Input: part model. Units: mm. Frame: model coordinates. A direction names the side the tool comes from. Coordinates: 2 decimals unless noted, no trailing zeros. Write each loop counter-clockwise with the first axis right and the second up, starting at its lowest first coordinate (ties: lowest second). Pieces come first, ordered by that corner, then holes.
from build123d import *

# Parameters (mm, degrees)
SKETCH1_W               = 40
SKETCH1_H               = 102
BOSS_EXTRUDE1_DEPTH     = 8.5
SKETCH2_W               = 35
SKETCH2_H               = 70
CUT_EXTRUDE1_DEPTH      = 3
SKETCH3_W               = 10.5
SKETCH3_H               = 10
CUT_EXTRUDE2_DEPTH      = 1.35
SKETCH4_W               = 12.5
SKETCH4_H               = 6
CUT_EXTRUDE3_DEPTH      = 3.1
SKETCH5_W               = 8.5
SKETCH5_H               = 17.5
PCB_PLACE_DEPTH         = 3.1
SKETCH6_W               = 8.5
SKETCH6_H               = 1.6
NICKEL_STRIP_HOLE_DEPTH = 66.369411807
CUT_EXTRUDE4_REACH      = 67.698
SKETCH7_W               = 8.5
SKETCH7_H               = 17.5
SKETCH8_W               = 8.5
SKETCH8_H               = 1.6
CUT_EXTRUDE5_DEPTH      = 10
SKETCH9_W               = 8.5
SKETCH9_H               = 102
NICKEL_STRIP_RAIL_DEPTH = 2.5
FILLET3_R               = 2.325
FILLET4_RADIUS          = 1.45
FILLET4_LENGTH          = 8.5


with BuildPart() as part:
    # Sketch1 → Boss-Extrude1 (new body)
    with BuildSketch(Plane(origin=(0, 0, 0), x_dir=(1, 0, 0), z_dir=(0, 1, 0))):
        with Locations((0, 11)):
            Rectangle(SKETCH1_W, SKETCH1_H)
    extrude(amount=BOSS_EXTRUDE1_DEPTH)

    # Sketch2 → Cut-Extrude1 (cut)
    with BuildSketch(Plane(origin=(0, 8.5, 0), x_dir=(1, 0, 0), z_dir=(0, 1, 0))):
        with Locations((0, -2)):
            Rectangle(SKETCH2_W, SKETCH2_H)
    extrude(amount=-CUT_EXTRUDE1_DEPTH, mode=Mode.SUBTRACT)

    # Sketch3 → Cut-Extrude2 (cut)
    with BuildSketch(Plane(origin=(0, 8.5, 0), x_dir=(1, 0, 0), z_dir=(0, 1, 0))):
        with Locations((-6.65, 38)):
            Rectangle(SKETCH3_W, SKETCH3_H)
        with Locations((6.65, 38)):
            Rectangle(SKETCH3_W, SKETCH3_H)
    extrude(amount=-CUT_EXTRUDE2_DEPTH, mode=Mode.SUBTRACT)

    # Sketch4 → Cut-Extrude3 (cut)
    with BuildSketch(Plane(origin=(0, 8.5, 0), x_dir=(1, 0, 0), z_dir=(0, 1, 0))):
        with Locations((6.65, 40)):
            Rectangle(SKETCH4_W, SKETCH4_H)
    extrude(amount=-CUT_EXTRUDE3_DEPTH, mode=Mode.SUBTRACT)

    # Sketch5 → PCB place (cut)
    with BuildSketch(Plane(origin=(0, 8.5, 0), x_dir=(1, 0, 0), z_dir=(0, 1, 0))):
        with Locations((6.65, 51.75)):
            Rectangle(SKETCH5_W, SKETCH5_H)
    extrude(amount=-PCB_PLACE_DEPTH, mode=Mode.SUBTRACT)

    # Sketch6 → Nickel strip hole (cut, through all)
    with BuildSketch(Plane(origin=(0, 5.4, 0), x_dir=(1, 0, 0), z_dir=(0, 1, 0))):
        with Locations((6.65, 59.7)):
            Rectangle(SKETCH6_W, SKETCH6_H)
    extrude(amount=-NICKEL_STRIP_HOLE_DEPTH, mode=Mode.SUBTRACT)

    # Cut-Extrude4: up to this face of the body (flat: up to its plane)
    cut_extrude4_end = Plane(part.part.faces().sort_by_distance((6.65, 5.4, -47.042077088))[0])
    # Sketch7 → Cut-Extrude4 (cut, up to the picked face)
    with BuildSketch(Plane(origin=(0, 8.5, 0), x_dir=(1, 0, 0), z_dir=(0, 1, 0)), mode=Mode.PRIVATE) as cut_extrude4_sk1:
        with Locations((-6.65, 51.75)):
            Rectangle(SKETCH7_W, SKETCH7_H)
    cut_extrude4_tool1 = split(extrude(cut_extrude4_sk1.sketch, amount=-CUT_EXTRUDE4_REACH, mode=Mode.PRIVATE), bisect_by=cut_extrude4_end, keep=Keep.BOTH, mode=Mode.PRIVATE)
    add(cut_extrude4_tool1.solids().sort_by(Axis((-6.65, 8.5, -51.75), (0, -1, 0)))[0], mode=Mode.SUBTRACT)

    # Sketch8 → Cut-Extrude5 (cut)
    with BuildSketch(Plane(origin=(0, 5.4, 0), x_dir=(1, 0, 0), z_dir=(0, 1, 0))):
        with Locations((-6.65, 43.8)):
            Rectangle(SKETCH8_W, SKETCH8_H)
    extrude(amount=-CUT_EXTRUDE5_DEPTH, mode=Mode.SUBTRACT)

    # Sketch9 → Nickel strip rail (cut)
    with BuildSketch(Plane.XZ):
        with Locations((-6.65, -11)):
            Rectangle(SKETCH9_W, SKETCH9_H)
        with Locations((6.65, -11)):
            Rectangle(SKETCH9_W, SKETCH9_H)
    extrude(amount=-NICKEL_STRIP_RAIL_DEPTH, mode=Mode.SUBTRACT)

    # Fillet3
    # the kernel refuses this fillet: 2.325 mm, written as the material it takes off along each edge
    with BuildSketch(Plane(origin=(3.4125, 7.15, -43), x_dir=(0, 0, 1), z_dir=(-1, 0, 0))) as fillet3_piece_1_section:
        with BuildLine():
            CenterArc((FILLET3_R, -FILLET3_R), FILLET3_R, 90, 90)
            Line((0, -FILLET3_R), (0, 0))
            Line((0, 0), (FILLET3_R, 0))
        make_face()
    fillet3_piece_1 = extrude(amount=20.125, mode=Mode.PRIVATE)
    fillet3_piece_1 = split(fillet3_piece_1, bisect_by=Plane(origin=(-11.9, 6.647157341, -42.474696814), z_dir=(1, 0, 0)), keep=Keep.TOP, mode=Mode.PRIVATE)
    fillet3_piece_1 = split(fillet3_piece_1, bisect_by=Plane(origin=(-1.4, 6.647157341, -42.474696814), z_dir=(-1, 0, 0)), keep=Keep.TOP, mode=Mode.PRIVATE)
    add(fillet3_piece_1, mode=Mode.SUBTRACT)
    with BuildSketch(Plane(origin=(-10.9, 2.5, -43), x_dir=(0, 1, 0), z_dir=(1, 0, 0))) as fillet3_piece_2:
        with BuildLine():
            CenterArc((FILLET3_R, FILLET3_R), FILLET3_R, 180, 90)
            Line((0, FILLET3_R), (0, 0))
            Line((0, 0), (FILLET3_R, 0))
        make_face()
    extrude(amount=8.5, mode=Mode.SUBTRACT)

    # Fillet4: full round fillet: the end face becomes a half cylinder, R = half its width
    fillet4_face = Plane((6.65, 3.95, -58.9), x_dir=(-1, 0, 0), z_dir=(0, 0, -1))  # on the end face: x along it, z out of the body
    fillet4_slab = fillet4_face.offset(-FILLET4_RADIUS / 2) * Box(FILLET4_LENGTH, 2 * FILLET4_RADIUS, FILLET4_RADIUS, mode=Mode.PRIVATE)  # the body's end, R deep
    fillet4_round = Plane((6.65, 3.95, -57.45), x_dir=(0, 0, -1), z_dir=(-1, 0, 0)) * Cylinder(FILLET4_RADIUS, FILLET4_LENGTH, mode=Mode.PRIVATE)  # its axis R under the face
    add(fillet4_slab - fillet4_round, mode=Mode.SUBTRACT)


solid = part.part
Item 1: Section query A-A, the plane x = 10. Return loops of the section in (y, z).
Item 2: Pull-direction query (Z, two-part tool) for faces 1 (the face through (0, 5, -62)), 2 (the face through (-16, 0, -12)), 3 (the face through (0, 5, 40)), 4 (the face through (-1.4, 8, -38)); classes: released by +Z, released by -Z, zero draft, split by the parting line, or undercut.
Item 3: Section query D-D, the plane x = -8. Return loops of the section in (y, z) (3 decimals).
Item 4: Material intervals for line 1 (X direction, y = 7.75, z = -38); line 2 (X direction, y = 6.5, z = -48.5); line 3 (Z direction, x = 6, y = 7), sorted ascending.
Item 5: Pin query (flat end, axial travel): pin 1 Ø1.2 at (x, z) = (8, -61.5) entering from -Y; pin 2 Ø2.5 at (x, z) = (-6, -56) entering from +Y; pin 3 Ø8 at (x, z) = (-10, 11.5) entering from +Y. Return the tip coordinate at first contact, or that it passes through.
Item 6: Access query for faces 5 (the face through (7, 6, -60.5)), 6 (the face through (10.9, 2, -23)), 7 (the face through (-7, 2.5, 0)), 8 (the face through (0, 5.5, 2)), 9 (the face through (15, 0, -12)). Directions: +Z, -Z, +X, -X, +Y, -Y. A direction counts if a zero-diameter tool reaches every point of the face in a straight line with its end or side. Return the directions, or none.
Item 7: Section query C-C, the plane z = -55. Return loops of the section in (x, y).
Item 8: Section query B-B, the plane y = 1.5. Return loops of the section in (x, z).
The answers:
1. outline: (2.5, -62) - (8.5, -62) - (8.5, -60.5) - (2.5, -60.5) - close; (2.5, -57.45) arc R1.45 ccw to (5.4, -57.45) - (5.4, -37) - (7.15, -37) - (7.15, -33) - (5.5, -33) - (5.5, 37) - (8.5, 37) - (8.5, 40) - (2.5, 40) - close
2. face 1: released by -Z
2. face 2: zero draft
2. face 3: released by +Z
2. face 4: undercut
3. outline: (2.5, -62) - (8.5, -62) - (8.5, -60.5) - (5.4, -60.5) - (5.4, -44.6) - (2.5, -44.6) - close; (2.5, -40.675) arc R2.325 ccw to (7.15, -40.675) - (7.15, -33) - (5.5, -33) - (5.5, 37) - (8.5, 37) - (8.5, 40) - (2.5, 40) - close
4. line 1: x = -20 to -11.9, -1.4 to 0.4, 12.9 to 20
4. line 2: x = -20 to -10.9, -2.4 to 2.4, 10.9 to 20
4. line 3: z = -62 to -60.5, -37 to -33, 37 to 40
5. pin 1: stops at y = 2.5
5. pin 2: stops at y = 5.4
5. pin 3: stops at y = 5.5
6. face 5: +Y, -Y
6. face 6: none
6. face 7: +Z, -Z, -Y
6. face 8: +Y
6. face 9: +Z, -Z, +X, -X, -Y
7. outline: (-20, 0) - (-10.9, 0) - (-10.9, 2.5) - (-2.4, 2.5) - (-2.4, 0) - (2.4, 0) - (2.4, 2.5) - (10.9, 2.5) - (10.9, 0) - (20, 0) - (20, 8.5) - (10.9, 8.5) - (10.9, 5.4) - (2.4, 5.4) - (2.4, 8.5) - (-2.4, 8.5) - (-2.4, 5.4) - (-10.9, 5.4) - (-10.9, 8.5) - (-20, 8.5) - close
8. outline: (-20, -62) - (-10.9, -62) - (-10.9, 40) - (-20, 40) - close; (-2.4, -62) - (2.4, -62) - (2.4, 40) - (-2.4, 40) - close; (10.9, -62) - (20, -62) - (20, 40) - (10.9, 40) - close
